Input: dimensioned drawing with shaded views. Units: mm. Origin: part minimum x, y, z. A direction names the side the tool comes from. Coordinates: 2 decimals unless noted, no trailing zeros. Loops run counter-clockwise (first coordinate to the right, second up) from the corner with the lowest first, then second, coordinate; pieces in that order, holes last.
(1) Mould query, pull axis X, two halves, no side actions, for the marked faces 1, 2, 3 and 4. Classes: released by +X, released by -X, zero draft, split by the parting line, or undercut.
(2) Set-up query: the marked faces 5 and 6. Return all of +Z, -Z, +X, -X, +Y, -Y with unobstructed straight access to the full face (end or side cutting, diameter ignored); none if empty.
(3) Section B-B, the plane z = 2.7. Return loops of the section in (x, y).
(4) Line query: L1, parallel to X at y = 11, z = 4.4 (1 decimal); L2, parallel to X at y = 31, z = 1.75 (1 decimal); L3, parallel to Y at x = 35, z = 3.15 (1 decimal). Output: solid intervals per line, ascending.
(5) Section A-A, the plane x = 34. Give the number of separate pieces and of enclosed holes in the cut face, then the cut area to 3 significant figures.
(6) Contact query for flat-ended pins moving along their axis: P1, Ø3, axis at x = 8, y = 10.5, coming from the +Z side; P2, Ø3, axis at x = 32.67, y = 32.36, coming from the -Z side. Output: stop coordinate, or through.
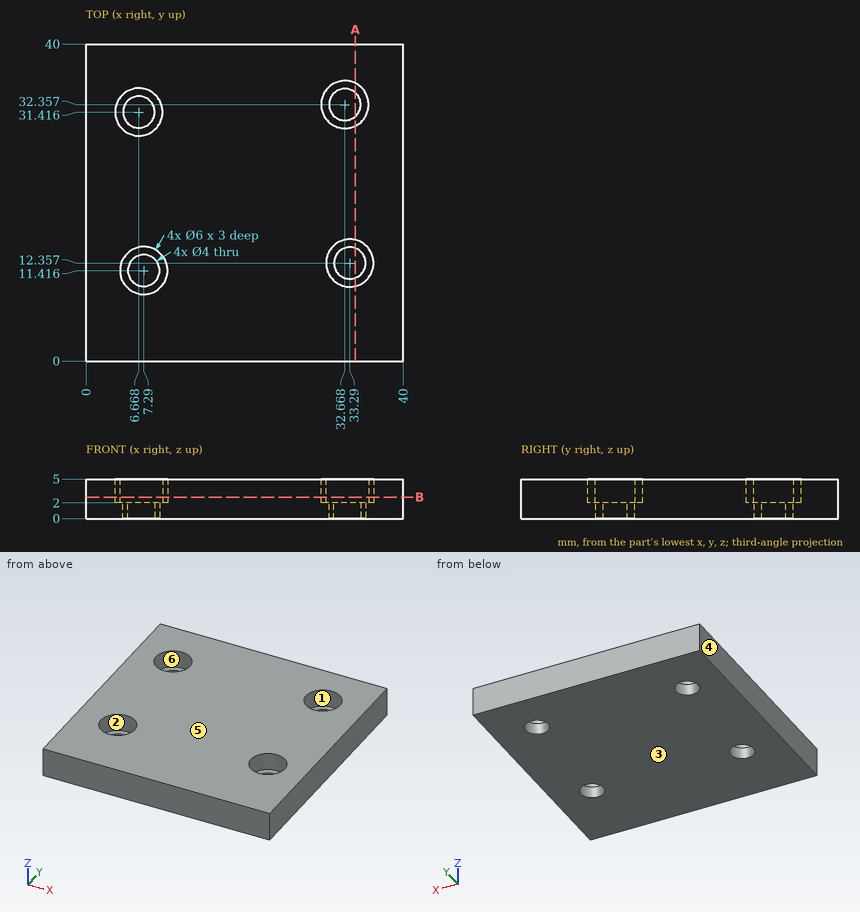
Report:
1. face 1: undercut
1. face 2: undercut
1. face 3: zero draft
1. face 4: released by -X
2. face 5: +Z, +X, -X, +Y, -Y
2. face 6: +Z
3. outline: (0, 0) - (40, 0) - (40, 40) - (0, 40) - close; hole circle Ø6 at (6.67, 31.42); hole circle Ø6 at (7.29, 11.42); hole circle Ø6 at (32.67, 32.36); hole circle Ø6 at (33.29, 12.36)
4. L1: x = 0 to 4.3, 10.3 to 30.6, 36 to 40
4. L2: x = 0 to 4.7, 8.6 to 31.2, 34.1 to 40
4. L3: y = 0 to 9.9, 14.8 to 30.5, 34.2 to 40
5. separate pieces: 3
5. enclosed holes: 0
5. area: 153 mm2
6. P1: stops at z = 2
6. P2: passes through
